```python
from build123d import *

# Parameters (mm, degrees)
SKETCH1_W           = 16.5
SKETCH1_H           = 9.7
BOSS_EXTRUDE1_DEPTH = 6.8
SKETCH2_W           = 16.5
SKETCH2_H           = 2
CUT_EXTRUDE1_DEPTH  = 5.8
CUT_EXTRUDE2_REACH  = 16.436
SKETCH3_R           = 2.75
CUT_EXTRUDE3_REACH  = 16.436
SKETCH4_R           = 2.4
SKETCH4_W           = 4.8
SKETCH4_H           = 2.9
SKETCH5_W           = 1.2
SKETCH5_H           = 2.5
SKETCH5_H_2         = 3.5
CUT_EXTRUDE4_DEPTH  = 12.739889267
BOSS_EXTRUDE2_DEPTH = 2
CHAMFER1_SIZE       = 1.8
FILLET4_R           = 2.5
SKETCH8_W           = 2.5
SKETCH8_H           = 9.5
SKETCH8_W_2         = 1.8
BOSS_EXTRUDE3_DEPTH = 1
BOSS_EXTRUDE5_DEPTH = 7
FILLET1_START       = -22
FILLET1_DEPTH       = 25.15
FILLET1_2_DEPTH     = 7.65
FILLET1_START_2     = -14.35
FILLET1_3_DEPTH     = 12
FILLET1_START_3     = -0.35
FILLET1_4_DEPTH     = 3.5
FILLET5_R           = 2


with BuildPart() as part:
    # Sketch1 → Boss-Extrude1 (new body)
    with BuildSketch(Plane(origin=(0, 0, 0), x_dir=(1, 0, 0), z_dir=(0, 1, 0))):
        Rectangle(SKETCH1_W, SKETCH1_H)
    extrude(amount=BOSS_EXTRUDE1_DEPTH)

    # Sketch2 → Cut-Extrude1 (cut)
    with BuildSketch(Plane(origin=(0, 6.8, 0), x_dir=(1, 0, 0), z_dir=(0, 1, 0))):
        with Locations((0, 1.35)):
            Rectangle(SKETCH2_W, SKETCH2_H)
    extrude(amount=-CUT_EXTRUDE1_DEPTH, mode=Mode.SUBTRACT)

    # Sketch3 → Cut-Extrude2 (cut, up to next)
    with BuildSketch(Plane(origin=(0, 0, -4.85), x_dir=(-1, 0, 0), z_dir=(0, 0, -1)), mode=Mode.PRIVATE) as cut_extrude2_sk1:
        with Locations((0, 3.9)):
            Circle(SKETCH3_R)
    cut_extrude2_tool1 = extrude(cut_extrude2_sk1.sketch, amount=-CUT_EXTRUDE2_REACH, mode=Mode.PRIVATE) & part.part
    # Sketch3 → Cut-Extrude2 (cut, up to next)
    with BuildSketch(Plane(origin=(0, 0, -4.85), x_dir=(-1, 0, 0), z_dir=(0, 0, -1)), mode=Mode.PRIVATE) as cut_extrude2_sk2:
        with BuildLine():
            Line((-2.75, 6.8), (-2.75, 3.9))
            ThreePointArc((-2.75, 3.9), (0, 6.65), (2.75, 3.9))
            Line((2.75, 3.9), (2.75, 6.8))
            Line((2.75, 6.8), (-2.75, 6.8))
        make_face()
    cut_extrude2_tool2 = extrude(cut_extrude2_sk2.sketch, amount=-CUT_EXTRUDE2_REACH, mode=Mode.PRIVATE) & part.part
    add(cut_extrude2_tool1.solids().sort_by_distance((0, 3.9, -4.85))[0], mode=Mode.SUBTRACT)
    add(cut_extrude2_tool2.solids().sort_by_distance((2.687823, 5.35, -4.85))[0], mode=Mode.SUBTRACT)

    # Sketch4 → Cut-Extrude3 (cut, up to next)
    with BuildSketch(Plane.XY.offset(4.85), mode=Mode.PRIVATE) as cut_extrude3_sk1:
        with Locations((0, 3.9)):
            Circle(SKETCH4_R)
    cut_extrude3_tool1 = extrude(cut_extrude3_sk1.sketch, amount=-CUT_EXTRUDE3_REACH, mode=Mode.PRIVATE) & part.part
    # Sketch4 → Cut-Extrude3 (cut, up to next)
    with BuildSketch(Plane.XY.offset(4.85), mode=Mode.PRIVATE) as cut_extrude3_sk2:
        with Locations((0, 5.35)):
            Rectangle(SKETCH4_W, SKETCH4_H)
    cut_extrude3_tool2 = extrude(cut_extrude3_sk2.sketch, amount=-CUT_EXTRUDE3_REACH, mode=Mode.PRIVATE) & part.part
    add(cut_extrude3_tool1.solids().sort_by_distance((0, 3.9, 4.85))[0], mode=Mode.SUBTRACT)
    add(cut_extrude3_tool2.solids().sort_by_distance((0, 5.35, 4.85))[0], mode=Mode.SUBTRACT)

    # Sketch5 → Cut-Extrude4 (cut, through all)
    with BuildSketch(Plane(origin=(0, 6.8, 0), x_dir=(1, 0, 0), z_dir=(0, 1, 0))):
        with Locations((-3.35, 3.6)):
            Rectangle(SKETCH5_W, SKETCH5_H)
        with Locations((3.35, 3.6)):
            Rectangle(SKETCH5_W, SKETCH5_H)
        with Locations((-3, -1.4)):
            Rectangle(SKETCH5_W, SKETCH5_H_2)
        with Locations((3, -1.4)):
            Rectangle(SKETCH5_W, SKETCH5_H_2)
    extrude(amount=-CUT_EXTRUDE4_DEPTH, mode=Mode.SUBTRACT)

    # Sketch7 → Boss-Extrude2 (add)
    with BuildSketch(Plane.XY.offset(-2.35)):
        Polygon((-6.35, 1), (-8.25, 2.9), (-8.25, 1), align=None)
        Polygon((8.25, 2.9), (8.25, 1), (6.35, 1), align=None)
    extrude(amount=BOSS_EXTRUDE2_DEPTH)

    # Chamfer1
    chamfer1_edges = [part.edges().sort_by_distance(p)[0] for p in [
        (-8.25, 6.8, -3.6),
        (8.25, 6.8, -3.6),
        (-8.25, 6.8, 2.25),
        (8.25, 6.8, 2.25),
    ]]
    chamfer(chamfer1_edges, length=CHAMFER1_SIZE)

    # Fillet4
    fillet4_edges = [part.edges().sort_by_distance(p)[0] for p in [
        (8.25, 2.5, 4.85),
        (-8.25, 2.5, 4.85),
    ]]
    fillet(fillet4_edges, radius=FILLET4_R)

    # Sketch8 → Boss-Extrude3 (add)
    # profile 1 of 7: a face of its own
    with BuildSketch(Plane.XZ):
        with Locations((-7, -9.6)):
            Rectangle(SKETCH8_W, SKETCH8_H)
    # profile 2 of 7: a face of its own
    with BuildSketch(Plane.XZ):
        with Locations((7, -9.6)):
            Rectangle(SKETCH8_W, SKETCH8_H)
    # profile 3 of 7: a face of its own
    with BuildSketch(Plane.XZ):
        with BuildLine():
            Line((8.25, -14.35), (5.75, -14.35))
            Line((5.75, -14.35), (5.75, -15.85))
            Line((5.75, -15.85), (7.25, -15.85))
            Line((7.25, -15.85), (7.25, -15.35))
            ThreePointArc((7.25, -15.35), (7.542893219, -14.642893219), (8.25, -14.35))
        make_face()
    # profile 4 of 7: a face of its own
    with BuildSketch(Plane.XZ):
        with BuildLine():
            Line((-7.25, -15.85), (-5.75, -15.85))
            Line((-5.75, -15.85), (-5.75, -14.35))
            Line((-5.75, -14.35), (-8.25, -14.35))
            ThreePointArc((-8.25, -14.35), (-7.542893219, -14.642893219), (-7.25, -15.35))
            Line((-7.25, -15.35), (-7.25, -15.85))
        make_face()
    # profile 5 of 7: a face of its own
    with BuildSketch(Plane.XZ):
        with BuildLine():
            Line((-5.75, -14.35), (-5.75, -15.85))
            Line((-5.75, -15.85), (-7.25, -15.85))
            Line((-7.25, -15.85), (-7.25, -18.85))
            ThreePointArc((-7.25, -18.85), (-6.517766953, -20.617766953), (-4.75, -21.35))
            Line((-4.75, -21.35), (4.75, -21.35))
            ThreePointArc((4.75, -21.35), (6.517766953, -20.617766953), (7.25, -18.85))
            Line((7.25, -18.85), (7.25, -15.85))
            Line((7.25, -15.85), (5.75, -15.85))
            Line((5.75, -15.85), (5.75, -14.35))
            Line((5.75, -14.35), (3.95, -14.35))
            Line((3.95, -14.35), (-3.95, -14.35))
            Line((-3.95, -14.35), (-5.75, -14.35))
        make_face()
        with BuildLine():
            ThreePointArc((-3.75, -18.85), (-4.75, -19.85), (-5.75, -18.85))
            Line((-5.75, -18.85), (-5.75, -15.85))
            ThreePointArc((-5.75, -15.85), (-4.75, -14.85), (-3.75, -15.85))
            Line((-3.75, -15.85), (-3.75, -18.85))
        make_face(mode=Mode.SUBTRACT)
        with BuildLine():
            ThreePointArc((3.75, -15.85), (4.75, -14.85), (5.75, -15.85))
            Line((5.75, -15.85), (5.75, -18.85))
            ThreePointArc((5.75, -18.85), (4.75, -19.85), (3.75, -18.85))
            Line((3.75, -18.85), (3.75, -15.85))
        make_face(mode=Mode.SUBTRACT)
    # profile 6 of 7: a face of its own
    with BuildSketch(Plane.XZ):
        with Locations((-4.85, -9.6)):
            Rectangle(SKETCH8_W_2, SKETCH8_H)
    # profile 7 of 7: a face of its own
    with BuildSketch(Plane.XZ):
        with Locations((4.85, -9.6)):
            Rectangle(SKETCH8_W_2, SKETCH8_H)
    extrude(amount=-BOSS_EXTRUDE3_DEPTH)

    # Sketch11 → Boss-Extrude5 (add)
    with BuildSketch(Plane(origin=(0, 0, -21.35), x_dir=(-1, 0, 0), z_dir=(0, 0, -1))):
        with BuildLine():
            Line((2.9, 1), (2.9, 3.9))
            ThreePointArc((2.9, 3.9), (2.050609665, 1.849390335), (0, 1))
            Line((0, 1), (2.9, 1))
        make_face()
        with BuildLine():
            ThreePointArc((0, 1), (-2.050609665, 1.849390335), (-2.9, 3.9))
            Line((-2.9, 3.9), (-2.9, 1))
            Line((-2.9, 1), (0, 1))
        make_face()
    extrude(amount=-BOSS_EXTRUDE5_DEPTH)

    # Fillet1: read off the stored shape, not the designer's step
    # Fillet1 outline → Fillet1 (cut)
    with BuildSketch(Plane.XY.offset(FILLET1_START)):
        with BuildLine():
            Line((-2.9, 3.9), (-2.9, 1.491681084))
            ThreePointArc((-2.9, 1.491681084), (-2.792530688, 1.801390075), (-2.516321365, 1.977962217))
            ThreePointArc((-2.516321365, 1.977962217), (-2.394047935, 2.033592906), (-2.261376801, 2.054662672))
            ThreePointArc((-2.261376801, 2.054662672), (-1.923333419, 2.208565025), (-1.572413793, 2.086849465))
            ThreePointArc((-1.572413793, 2.086849465), (-2.183322366, 2.903454242), (-2.4, 3.9))
            Line((-2.4, 3.9), (-2.4, 2.557427842))
            ThreePointArc((-2.4, 2.557427842), (-2.661061818, 3.206278154), (-2.75, 3.9))
            Line((-2.75, 3.9), (-2.75, 2.979402368))
            ThreePointArc((-2.75, 2.979402368), (-2.862254356, 3.433631047), (-2.9, 3.9))
        make_face()
        with BuildLine():
            ThreePointArc((2.4, 3.9), (2.183322366, 2.903454242), (1.572413793, 2.086849465))
            ThreePointArc((1.572413793, 2.086849465), (1.923333419, 2.208565025), (2.261376801, 2.054662672))
            ThreePointArc((2.261376801, 2.054662672), (2.394047935, 2.033592906), (2.516321365, 1.977962217))
            ThreePointArc((2.516321365, 1.977962217), (2.792530688, 1.801390075), (2.9, 1.491681084))
            Line((2.9, 1.491681084), (2.9, 3.9))
            ThreePointArc((2.9, 3.9), (2.862254356, 3.433631047), (2.75, 2.979402368))
            Line((2.75, 2.979402368), (2.75, 3.9))
            ThreePointArc((2.75, 3.9), (2.661061818, 3.206278154), (2.4, 2.557427842))
            Line((2.4, 2.557427842), (2.4, 3.9))
        make_face()
    extrude(amount=FILLET1_DEPTH, mode=Mode.SUBTRACT)

    # Fillet1 2 outline → Fillet1 2 (cut)
    with BuildSketch(Plane.XY.offset(FILLET1_START)):
        with BuildLine():
            ThreePointArc((-2.516321365, 1.977962217), (-2.264497484, 1.97297005), (-2.047058824, 1.845845631))
            ThreePointArc((-2.047058824, 1.845845631), (-2.150447744, 1.954344712), (-2.248093276, 2.068040224))
            ThreePointArc((-2.248093276, 2.068040224), (-2.254798094, 2.06141406), (-2.261376801, 2.054662672))
            ThreePointArc((-2.261376801, 2.054662672), (-2.394047935, 2.033592906), (-2.516321365, 1.977962217))
        make_face()
        with BuildLine():
            ThreePointArc((2.047058824, 1.845845631), (2.264497484, 1.97297005), (2.516321365, 1.977962217))
            ThreePointArc((2.516321365, 1.977962217), (2.394047935, 2.033592906), (2.261376801, 2.054662672))
            ThreePointArc((2.261376801, 2.054662672), (2.254798094, 2.06141406), (2.248093276, 2.068040224))
            ThreePointArc((2.248093276, 2.068040224), (2.150447744, 1.954344712), (2.047058824, 1.845845631))
        make_face()
    extrude(amount=FILLET1_2_DEPTH, mode=Mode.SUBTRACT)

    # Fillet1 3 outline → Fillet1 3 (cut)
    with BuildSketch(Plane.XY.offset(FILLET1_START_2)):
        with BuildLine():
            ThreePointArc((-2.516321365, 1.977962217), (-2.641945637, 1.929245147), (-2.75, 1.848752506))
            Line((-2.75, 1.848752506), (-2.75, 1.55479212))
            ThreePointArc((-2.75, 1.55479212), (-2.687698916, 1.796493711), (-2.516321365, 1.977962217))
        make_face()
        with BuildLine():
            ThreePointArc((-2.261376801, 2.054662672), (-2.068743309, 2.020781403), (-1.903846154, 1.915593332))
            ThreePointArc((-1.903846154, 1.915593332), (-2.01831936, 2.032143753), (-2.125669903, 2.155285851))
            ThreePointArc((-2.125669903, 2.155285851), (-2.197803986, 2.1107474), (-2.261376801, 2.054662672))
        make_face()
        with BuildLine():
            ThreePointArc((2.261376801, 2.054662672), (2.197803986, 2.1107474), (2.125669903, 2.155285851))
            ThreePointArc((2.125669903, 2.155285851), (2.01831936, 2.032143753), (1.903846154, 1.915593332))
            ThreePointArc((1.903846154, 1.915593332), (2.068743309, 2.020781403), (2.261376801, 2.054662672))
        make_face()
        with BuildLine():
            ThreePointArc((2.75, 1.848752506), (2.641945637, 1.929245147), (2.516321365, 1.977962217))
            ThreePointArc((2.516321365, 1.977962217), (2.687698916, 1.796493711), (2.75, 1.55479212))
            Line((2.75, 1.55479212), (2.75, 1.848752506))
        make_face()
    extrude(amount=FILLET1_3_DEPTH, mode=Mode.SUBTRACT)

    # Fillet1 4 outline → Fillet1 4 (cut)
    with BuildSketch(Plane.XY.offset(FILLET1_START_3)):
        with BuildLine():
            Line((-2.4, 2.031761721), (-2.4, 1.70910977))
            ThreePointArc((-2.4, 1.70910977), (-2.364051937, 1.895270453), (-2.261376801, 2.054662672))
            ThreePointArc((-2.261376801, 2.054662672), (-2.331496818, 2.048105681), (-2.4, 2.031761721))
        make_face()
        with BuildLine():
            ThreePointArc((2.261376801, 2.054662672), (2.364051937, 1.895270453), (2.4, 1.70910977))
            Line((2.4, 1.70910977), (2.4, 2.031761721))
            ThreePointArc((2.4, 2.031761721), (2.331496818, 2.048105681), (2.261376801, 2.054662672))
        make_face()
    extrude(amount=FILLET1_4_DEPTH, mode=Mode.SUBTRACT)

    # Fillet5
    fillet5_edges = [part.edges().sort_by_distance(p)[0] for p in [
        (-3.95, 0.5, -14.35),
        (3.95, 0.5, -14.35),
        (6.1, 1, -4.85),
        (-6.1, 1, -4.85),
    ]]
    fillet(fillet5_edges, radius=FILLET5_R)


solid = part.part
```
Check sheet for the modelled part. Datum: model origin and axes. Units: mm. A direction names the side the tool comes from. Coordinates: 2 decimals unless noted, no trailing zeros. Loops run counter-clockwise (first coordinate to the right, second up) from the corner with the lowest first, then second, coordinate; pieces in that order, holes last.
1) Material ranges on probe 1 along Z at (x, y) = (5.25, 4.25); probe 2 along X at (y, z) = (0.5, -15.75); probe 3 along X at (y, z) = (0.5, -9.5), recorded low to high.
2) Sectioned sample at D-D (y = 4.5). Record the boundary of the cut face in (x, z), and give its area (3 significant figures).
3) Sectioned sample at B-B (y = 6). Record the boundary of the cut face in (x, z), and give its area (3 significant figures).
4) Gauge pin test, flat ends, axial feed: pin 1 (1.1 mm diameter, centred on y = 0.5, z = -17.5, fed in from +X); pin 2 (1.9 mm diameter, centred on x = 7, y = 4, fed in from -Z); pin 3 (0.8 mm diameter, centred on y = 0.5, z = -17, fed in from -X); pin 4 (1.5 mm diameter, centred on x = 0, y = 5, fed in from +Z). Record the tip position at first contact, or that the pin passes through.
5) Release check for a two-part mould opening along Z. For faces 1 (the face through (-7.34, 5.91, -3.58)), 2 (the face through (-6.07, 1.57, -5.45)), 3 (the face through (3, 3, 3.15)) record: released by +Z, released by -Z, zero draft, split by the parting line, or undercut.
6) Sectioned sample at C-C (x = 1). Record the boundary of the cut face in (y, z).
7) Access from +Z, -Z, +X, -X, +Y, -Y to the whole of each face (thin tool, end or side, straight path). Record for faces 4 (the face through (2.4, 5, 4)), 5 (the face through (-4.77, 0.49, -14.85)), 6 (the face through (-7.25, 0.5, -17.1)).
8) Sectioned sample at A-A (z = -16.5). Record the boundary of the cut face in (x, y).
Check sheet entries:
1. probe 1: z = -4.85 to -2.35, -0.35 to 4.85
1. probe 2: x = -7.25 to -5.74, -3.76 to 3.76, 5.74 to 7.25
1. probe 3: x = -8.25 to -3.95, 3.95 to 8.25
2. outline: (-8.25, -4.85) - (-3.95, -4.85) - (-3.95, -2.35) - (-8.25, -2.35) - close; (-8.25, -0.35) - (-3.6, -0.35) - (-3.6, 3.15) - (-2.4, 3.15) - (-2.4, 4.85) - (-5.75, 4.85) arc R2.5 ccw to (-8.25, 2.35) - close; (2.4, 3.15) - (3.6, 3.15) - (3.6, -0.35) - (8.25, -0.35) - (8.25, 2.35) arc R2.5 ccw to (5.75, 4.85) - (2.4, 4.85) - close; (3.95, -4.85) - (8.25, -4.85) - (8.25, -2.35) - (3.95, -2.35) - close
2. area: 71.3 mm2
3. outline: (-7.25, -4.85) - (-3.95, -4.85) - (-3.95, -2.35) - (-7.25, -2.35) - close; (-7.25, -0.35) - (-3.6, -0.35) - (-3.6, 3.15) - (-2.4, 3.15) - (-2.4, 4.85) - (-5.75, 4.85) arc R2.5 ccw to (-7.25, 4.35) - close; (2.4, 3.15) - (3.6, 3.15) - (3.6, -0.35) - (7.25, -0.35) - (7.25, 4.35) arc R2.5 ccw to (5.75, 4.85) - (2.4, 4.85) - close; (3.95, -4.85) - (7.25, -4.85) - (7.25, -2.35) - (3.95, -2.35) - close
3. area: 58.1 mm2
4. pin 1: stops at x = 7.25
4. pin 2: stops at z = -4.85
4. pin 3: stops at x = -7.25
4. pin 4: passes through
5. face 1: zero draft
5. face 2: released by -Z
5. face 3: undercut
6. outline: (0, -21.35) - (1.18, -21.35) - (1.18, -14.35) - (0, -14.35) - close; (0, -4.85) - (1.34, -4.85) - (1.34, -2.35) - (1, -2.35) - (1, -0.35) - (1.72, -0.35) - (1.72, 4.85) - (0, 4.85) - close
7. face 4: +Z, -Z, +Y
7. face 5: +Y, -Y
7. face 6: -Z, -X, +Y, -Y
8. outline: (-7.25, 0) - (-5.75, 0) - (-5.75, 1) - (-7.25, 1) - close; (-3.75, 0) - (3.75, 0) - (3.75, 1) - (2.9, 1) - (2.9, 1.49) arc R0.5 ccw to (2.05, 1.85) arc R2.9 cw to (-2.05, 1.85) arc R0.5 ccw to (-2.9, 1.49) - (-2.9, 1) - (-3.75, 1) - close; (5.75, 0) - (7.25, 0) - (7.25, 1) - (5.75, 1) - close
